Here's how the part is built. I have some questions about the finished solid (model axes, mm). A direction names the side the tool comes from. Round coordinates to 2 decimals unless told otherwise and drop trailing zeros. Order: outer loops, then holes, each group sorted by start corner. A loop starts at its lowest first (then second) coordinate and runs counter-clockwise, first axis right, second up. Notation, with made-up numbers: (43, -24) - (91, -24) arc R21 ccw to (91, -18) - close; hole circle Ø8 at (77.5, -34). An arc over 180 degrees is marked (long way). Answer as a JSON object with one key per item and string values.
```python
from build123d import *

# Parameters (mm, degrees)
SKETCH1_R                                            = 3.175
SKETCH1_R_2                                          = 1.524
BOSS_EXTRUDE1_DEPTH                                  = 125
SKETCH2_R                                            = 1.38938
F_5_40_HOLE_FOR_SET_SCREW_ATTACHING_SHAFT_DEPTH      = 10
F_5_40_HOLE_FOR_SET_SCREW_ATTACHING_SHAFT_DEPTH_BACK = 10
SKETCH3_W                                            = 25
SKETCH3_H                                            = 14.833516594
CUT_EXTRUDE2_DEPTH                                   = 4.175000101
SKETCH4_R                                            = 0.889
CUT_EXTRUDE3_DEPTH                                   = 3


with BuildPart() as part:
    # Sketch1 → Boss-Extrude1 (new body)
    with BuildSketch(Plane(origin=(0, 0, 0), x_dir=(0, 0, -1), z_dir=(1, 0, 0))):
        Circle(SKETCH1_R)
        Circle(SKETCH1_R_2, mode=Mode.SUBTRACT)
    extrude(amount=BOSS_EXTRUDE1_DEPTH)

    # Sketch2 → 5-40 hole for set screw attaching shaft (cut, two sides)
    with BuildSketch(Plane.XY) as f_5_40_hole_for_set_screw_attaching_shaft_sk:
        with Locations((4.171703898, 0)):
            Circle(SKETCH2_R)
    extrude(amount=F_5_40_HOLE_FOR_SET_SCREW_ATTACHING_SHAFT_DEPTH, mode=Mode.SUBTRACT)
    extrude(f_5_40_hole_for_set_screw_attaching_shaft_sk.sketch, amount=-F_5_40_HOLE_FOR_SET_SCREW_ATTACHING_SHAFT_DEPTH_BACK, mode=Mode.SUBTRACT)

    # Sketch3 → Cut-Extrude2 (cut, through all)
    with BuildSketch(Plane.XY):
        with Locations((32.5, -1.779757755)):
            Rectangle(SKETCH3_W, SKETCH3_H)
    extrude(amount=CUT_EXTRUDE2_DEPTH, mode=Mode.SUBTRACT)

    # Sketch4 → Cut-Extrude3 (cut)
    with BuildSketch(Plane.XY):
        with Locations((30.5963642, 0)):
            Circle(SKETCH4_R)
    extrude(amount=-CUT_EXTRUDE3_DEPTH, mode=Mode.SUBTRACT)


solid = part.part
```
1. Imagine slicing it at A-A (x = 72.5). List the corners of the cut face in (y, z) for me (3 decimals), plus the area to 3 significant figures.
Responses:
{"outline": "circle Ø6.35 at (0, 0); hole circle Ø3.048 at (0, 0)", "area": "24.4 mm2"}
2. If I drill on L1, parallel to X at y = 0, z = -2.5; L2, parallel to X at y = 0.5, z = -2.5; L3, parallel to Z at x = 77, y = 0.25, over which ranges is the centre line in solid material (lowest first)? Write a range as [from, to].
Responses:
{"L1": "[0, 2.78], [5.56, 29.71], [31.49, 125]", "L2": "[0, 2.88], [5.47, 29.86], [31.33, 125]", "L3": "[-3.17, -1.5], [1.5, 3.17]"}
3. For P1, Ø0.5, axis at x = 30, y = 2.5, coming from the +Z side; P2, Ø1.4, axis at x = 30.5, y = 0, coming from the +Z side; P3, Ø1.5, axis at x = 77.5, z = -1, coming from the -Y side, each with a flat end and sliding along its axis, tell me the tip position at first contact or that it passes through.
Responses:
{"P1": "z = 0", "P2": "z = -3", "P3": "y = -3.17"}
4. Imagine slicing it at B-B (x = 36). List the corners of the cut face in (y, z) for me (3 decimals), plus the area to 3 significant figures.
Responses:
{"outline": "(-3.175, 0) arc R3.175 ccw to (3.175, 0) - (1.524, 0) arc R1.524 cw to (-1.524, 0) - close", "area": "12.2 mm2"}
5. For faces 1 (the face through (2.784, 0.061, -2.166)), 2 (the face through (20, 0, 2)), which set-ups out of +Z, -Z, +X, -X, +Y, -Y let a thin tool reach every point of the face, with its end or its side?
Responses:
{"face 1": "+Z, -Z", "face 2": "+Z, +Y, -Y"}
6. Thinking about a two-plate mould opening in X: for faces 3 (the face through (45, 0, 2)), 4 (the face through (0, 1.5, 0.8)), 5 (the face through (125, 1.5, 0.8)), 6 (the face through (61.625, 0.458, -1.454)), which applies, pulls with the +X half, pulls with the -X half, needs draft (parallel to the pull), parting line crosses it, or undercut?
Responses:
{"face 3": "undercut", "face 4": "pulls with the -X half", "face 5": "pulls with the +X half", "face 6": "needs draft"}
